```python
from build123d import *

# Parameters (mm, degrees)
F1_DEPTH = 6.35
F2_R     = 3.175
F3_DEPTH = 25.4
F4_R     = 3.175
F5_DEPTH = 2.54
F6_SIZE  = 2.54


with BuildPart() as f1:
    # F0 (on Front) → F1 (new body)
    with BuildSketch(Plane.XZ):
        with BuildLine():
            ThreePointArc((19.05, 25.4), (17.1901280605, 29.8901280605), (12.7, 31.75))
            Line((12.7, 31.75), (-12.7, 31.75))
            ThreePointArc((-12.7, 31.75), (-17.1901280605, 29.8901280605), (-19.05, 25.4))
            Line((-19.05, 25.4), (-19.05, -25.4))
            ThreePointArc((-19.05, -25.4), (-17.1901280605, -29.8901280605), (-12.7, -31.75))
            Line((-12.7, -31.75), (12.7, -31.75))
            ThreePointArc((12.7, -31.75), (17.1901280605, -29.8901280605), (19.05, -25.4))
            Line((19.05, -25.4), (19.05, 25.4))
        make_face()
    extrude(amount=F1_DEPTH)

    # F2 (on face) → F3 (cut)
    with BuildSketch(Plane.XZ.offset(6.35)):
        Circle(F2_R)
    extrude(amount=-F3_DEPTH, mode=Mode.SUBTRACT)

    # F4 (on face) → F5 (join)
    with BuildSketch(Plane.XZ.offset(6.35)):
        with BuildLine():
            ThreePointArc((-12.319, 30.099), (-15.9111024484, 28.6111024484), (-17.399, 25.019))
            Line((-17.399, 25.019), (-17.399, -25.019))
            ThreePointArc((-17.399, -25.019), (-15.9111024484, -28.6111024484), (-12.319, -30.099))
            Line((-12.319, -30.099), (12.319, -30.099))
            ThreePointArc((12.319, -30.099), (15.9111024484, -28.6111024484), (17.399, -25.019))
            Line((17.399, -25.019), (17.399, 25.019))
            ThreePointArc((17.399, 25.019), (15.9111024484, 28.6111024484), (12.319, 30.099))
            Line((12.319, 30.099), (-12.319, 30.099))
        make_face()
        Circle(F4_R, mode=Mode.SUBTRACT)
    extrude(amount=F5_DEPTH)

    # F6
    f6_edges = [f1.edges().sort_by_distance(p)[0] for p in [
        (-19.05, 0, 0),
    ]]
    chamfer(f6_edges, length=F6_SIZE)


solid = f1.part
```
The model under review builds one solid part; all positions refer to its coordinate system, in mm. A direction names the side the tool comes from. Round coordinates to 2 decimals unless told otherwise and drop trailing zeros. Order: outer loops, then holes, each group sorted by start corner. A loop starts at its lowest first (then second) coordinate and runs counter-clockwise, first axis right, second up.
Item 1: Add section C-C, the plane y = -5.5. State the section outline as (x, z) points (3 decimals), and give its area (3 significant figures).
Working result:
outline: (-19.05, -25.4) arc R6.35 ccw to (-12.7, -31.75) - (12.7, -31.75) arc R6.35 ccw to (19.05, -25.4) - (19.05, 25.4) arc R6.35 ccw to (12.7, 31.75) - (-12.7, 31.75) arc R6.35 ccw to (-19.05, 25.4) - close; hole circle Ø6.35 at (0, 0)
area: 2,350 mm2
Item 2: For pin 1 (4 mm diameter, centred on x = 0, z = 0, fed in from -Y); pin 2 (2 mm diameter, centred on x = 2, y = -7.5, fed in from +Z); pin 3 (1.5 mm diameter, centred on y = -1.5, z = -20.5, fed in from +X); pin 4 (2 mm diameter, centred on y = -8, z = 12.5, fed in from +X), all flat-tipped, find the tip position at first contact; note any pin that passes through.
Working result:
pin 1: passes through
pin 2: stops at z = 30.1
pin 3: stops at x = 18.76
pin 4: stops at x = 17.4
Item 3: To check wall thickness, follow probe 1 along Z at (x, y) = (0, -3.5) (3 decimals); probe 2 along X at (y, z) = (-7.25, 9); probe 3 along Z at (x, y) = (1.5, -6). State the ranges of each line that lie inside material, in increasing order.
Working result:
probe 1: z = -31.75 to -3.175, 3.175 to 31.75
probe 2: x = -17.4 to 17.4
probe 3: z = -31.75 to -2.8, 2.8 to 31.75
Item 4: Add section B-B, the plane z = 0. State the section outline as (x, y) points (3 decimals), and give its area (3 significant figures).
Working result:
outline: (-19.05, -6.35) - (-17.399, -6.35) - (-17.399, -8.89) - (-3.175, -8.89) - (-3.175, 0) - (-16.51, 0) - (-19.05, -2.54) - close; (3.175, -8.89) - (17.399, -8.89) - (17.399, -6.35) - (19.05, -6.35) - (19.05, -2.54) - (16.51, 0) - (3.175, 0) - close
area: 267 mm2
Item 5: Add section D-D, the plane x = -4. State the section outline as (y, z) points.
Working result:
outline: (-8.89, -30.1) - (-6.35, -30.1) - (-6.35, -31.75) - (-2.54, -31.75) - (0, -29.21) - (0, 29.21) - (-2.54, 31.75) - (-6.35, 31.75) - (-6.35, 30.1) - (-8.89, 30.1) - close
Item 6: Add section A-A, the plane x = 0. State the section outline as (y, z) points (3 decimals), and give its area (3 significant figures).
Working result:
outline: (-8.89, -30.099) - (-6.35, -30.099) - (-6.35, -31.75) - (-2.54, -31.75) - (0, -29.21) - (0, -3.175) - (-8.89, -3.175) - close; (-8.89, 3.175) - (0, 3.175) - (0, 29.21) - (-2.54, 31.75) - (-6.35, 31.75) - (-6.35, 30.099) - (-8.89, 30.099) - close
area: 493 mm2
Item 7: Machinability: for faces 1 (the flat face through (17.399, -8, 0)), 2 (the flat face through (-17.399, -8, 0)), 3 (the flat face through (0, -8, 30.099)), 4 (the cylindrical face through (15.87, -7.6, -28.65)), 5 (the flat face through (-0.18, -1.25, -30.46)), which of the approach directions +Z, -Z, +X, -X, +Y, -Y give a long, thin tool a straight path to every point of the face, cutting with its end or side? Answer none if there is none.
Working result:
face 1: +Z, -Z, +X, -Y
face 2: +Z, -Z, -X, -Y
face 3: +Z, +X, -X, -Y
face 4: -Z, +X, -Y
face 5: -Z, +X, -X, +Y
